Design review of the part shown in the three views and the two pictorial views. Dimensions are in mm from the part's minimum x, y and z. A direction names the side the tool comes from. Round coordinates to 2 decimals unless told otherwise and drop trailing zeros. Write each loop counter-clockwise with the first axis right and the second up, starting at its lowest first coordinate (ties: lowest second). Pieces come first, ordered by that corner, then holes. Notation, with made-up numbers: (88.5, 76.25) - (96.5, 76.25) arc R18 cw to (96.5, 105.25) - close; hole circle Ø6 at (-4, 80.25). An arc over 180 degrees is marked (long way). One line per item, written item: value. Start each with the question number.
Q1. For probe 1 along X at (y, z) = (3, 18); probe 2 along Z at (x, y) = (81, 11); probe 3 along X at (y, z) = (1.5, 35), list the stretches that pass through material, from the lowest coordinate up.
Q2. Mouldability with a two-part tool opening along Z and no side actions: class the marked faces 3, 4, 5 and 6 as +Z half, -Z half, draft (parallel to the pull), parting line (faces both ways), or undercut.
Q3. Clearance check with a flat-ended pin moving along its axis: pin 1 Ø2 at (x, z) = (7.05, 38.87) entering from +Y (1 decimal). State where the tip first meets the part, or that it passes through.
Q4. Add section A-A on x = 53.5. Write out the cut boundary in (y, z).
Q5. Tool access review of the marked faces 1 and 2: name each direction out of +Z, -Z, +X, -X, +Y, -Y from which nothing blocks a thin tool from reaching the whole face with its end or side.
Q6. Add section B-B on y = 6. Write out the cut boundary in (x, z).
Q7. Add section C-C on z = 44. Write out the cut boundary in (x, y), and give its area (3 significant figures).
Q8. Add section D-D on x = 69.5. Write out the cut boundary in (y, z), and give its area (3 significant figures).
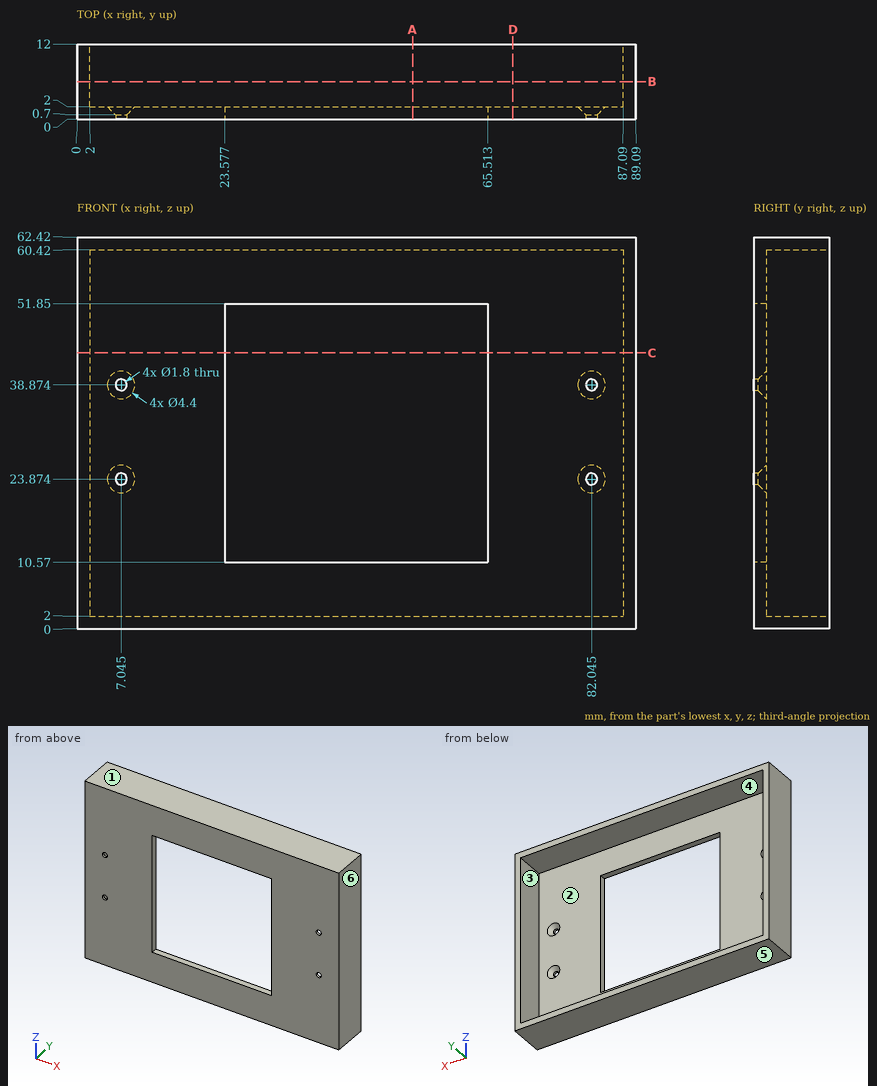
Result set:
1. probe 1: x = 0 to 2, 87.09 to 89.09
1. probe 2: z = 0 to 2, 60.42 to 62.42
1. probe 3: x = 0 to 23.58, 65.51 to 89.09
2. face 3: undercut
2. face 4: undercut
2. face 5: -Z half
2. face 6: draft
3. pin 1: stops at y = 0.8
4. outline: (0, 0) - (12, 0) - (12, 2) - (2, 2) - (2, 10.57) - (0, 10.57) - close; (0, 51.85) - (2, 51.85) - (2, 60.42) - (12, 60.42) - (12, 62.42) - (0, 62.42) - close
5. face 1: +Z, +X, -X, +Y, -Y
5. face 2: +Y
6. outline: (0, 0) - (89.09, 0) - (89.09, 62.42) - (0, 62.42) - close; hole (2, 2) - (87.09, 2) - (87.09, 60.42) - (2, 60.42) - close
7. outline: (0, 0) - (23.58, 0) - (23.58, 2) - (2, 2) - (2, 12) - (0, 12) - close; (65.51, 0) - (89.09, 0) - (89.09, 12) - (87.09, 12) - (87.09, 2) - (65.51, 2) - close
7. area: 134 mm^2
8. outline: (0, 0) - (12, 0) - (12, 2) - (2, 2) - (2, 60.42) - (12, 60.42) - (12, 62.42) - (0, 62.42) - close
8. area: 165 mm^2
